Geometry check sheet. Reference: drawing and pictorial views, mm from the part's lowest x, y, z. A direction names the side the tool comes from. Round coordinates to 2 decimals unless told otherwise and drop trailing zeros. Write each loop counter-clockwise with the first axis right and the second up, starting at its lowest first coordinate (ties: lowest second). Pieces come first, ordered by that corner, then holes. Notation, with made-up numbers: (64.25, 38) -> (80.25, 38) arc R28 ccw to (80.25, 60) -> close; hole circle Ø10 at (-36, 9). An arc over 180 degrees is marked (long way). Answer as a JSON object with one key per item and string values. Group by question number.
(1) Sectioned sample at A-A on y = 4. Record the cut outline in (x, z) (1 decimal).
(2) Set-up check for the marked faces 4, 5, 6, 7 and 8: record each of +Z, -Z, +X, -X, +Y, -Y from which the full face is reachable in a straight line by a thin tool's end or side.
(3) Draft check along X on the marked faces 1, 2 and 3. Enter one of: released by +X, released by -X, zero draft, split by the parting line, or undercut.
(4) Scan lines: L1, parallel to X at y = 6.5, z = 14 (1 decimal); L2, parallel to Z at x = 16.5, y = 6.5; L3, parallel to Z at x = 31.5, y = 2.75. Record each from-to range of solid material in increasing order. Write a range as from..to.
(5) Gauge pin test, flat ends, axial feed: pin 1 Ø1.4 at (x, z) = (10.5, 20.5) entering from -Y; pin 2 Ø1.4 at (x, z) = (24, 21) entering from -Y; pin 3 Ø5 at (x, y) = (4, 16) entering from +Z; pin 4 Ø8 at (x, z) = (16.5, 22.5) entering from +Y (1 decimal). Record the tip position at first contact, or that the pin passes through.
(6) Sectioned sample at D-D on x = 31. Record the cut outline in (y, z).
(7) Sectioned sample at B-B on z = 15. Record the cut outline in (x, y) (1 decimal).
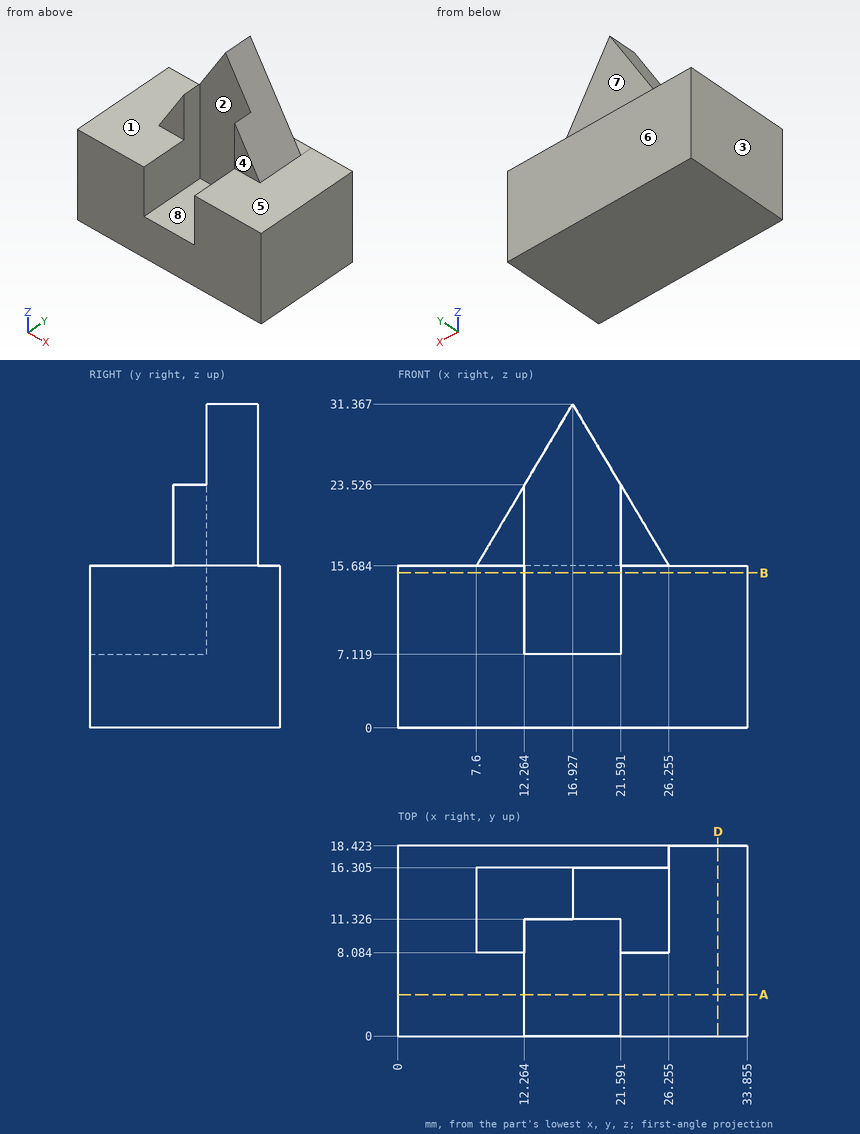
Computed values:
{
 "1": {"outline": "(0, 0) -> (33.9, 0) -> (33.9, 15.7) -> (21.6, 15.7) -> (21.6, 7.1) -> (12.3, 7.1) -> (12.3, 15.7) -> (0, 15.7) -> close"},
 "2": {"face 4": "+Z, +X, -X, -Y", "face 5": "+Z, +X, -Y", "face 6": "+Z, -Z, +X, -X, +Y", "face 7": "+Z, +X, -X, +Y", "face 8": "+Z, -Y"},
 "3": {"face 1": "zero draft", "face 2": "undercut", "face 3": "released by -X"},
 "4": {"L1": "0..12.3, 21.6..33.9", "L2": "0..7.12", "L3": "0..15.68"},
 "5": {"pin 1": "y = 8.08", "pin 2": "through", "pin 3": "z = 15.68", "pin 4": "y = 16.3"},
 "6": {"outline": "(0, 0) -> (18.42, 0) -> (18.42, 15.68) -> (0, 15.68) -> close"},
 "7": {"outline": "(0, 0) -> (12.3, 0) -> (12.3, 11.3) -> (21.6, 11.3) -> (21.6, 0) -> (33.9, 0) -> (33.9, 18.4) -> (0, 18.4) -> close"}
}
